Geometry check sheet. Reference: the model listing, model coordinates, mm. Face numbers are marked on the shaded views. Coordinates: 2 decimals unless noted, no trailing zeros. Loops run counter-clockwise (first coordinate to the right, second up) from the corner with the lowest first, then second, coordinate; pieces in that order, holes last. Notation, with made-up numbers: (69, -9.5) -> (76, -9.5) arc R13 ccw to (76, 2.5) -> close; hole circle Ø1 at (74.5, 63.25). An arc over 180 degrees is marked (long way). Answer as a JSON object with one key per item and string values.
from build123d import *

# Parameters (mm, degrees)
SKETCH2_W          = 5.4
SKETCH2_H          = 3.175
CUT_EXTRUDE1_DEPTH = 2
SKETCH4_R          = 2.7
CUT_EXTRUDE2_DEPTH = 3.175


with BuildPart() as part:
    # Sketch1 → Revolve3 (revolve)
    with BuildSketch(Plane(origin=(0, 0, 0), x_dir=(0, 0, -1), z_dir=(1, 0, 0))):
        with BuildLine():
            Line((4, 1.352218356), (4, 6.017854764))
            Line((4, 6.017854764), (0, 6.017854764))
            Line((0, 6.017854764), (0, -2.176614275))
            add(Edge.make_bspline(
                [(0, -2.176614275), (6.891187287, -2.176614275), (4.190169576, 0.853129288)],
                knots=[1.570796327, 1.570796327, 1.570796327, 3.544345546, 3.544345546, 3.544345546], degree=2, weights=[1, 0.551383512, 1]))
            ThreePointArc((4.190169576, 0.853129288), (4.049153077, 1.085172309), (4, 1.352218356))
        make_face()
    revolve(axis=Axis((0, 6.017854764, 0), (0, 1, 0)))

    # Sketch2 → Cut-Extrude1 (cut)
    with BuildSketch(Plane(origin=(0, 6.017854764, 0), x_dir=(1, 0, 0), z_dir=(0, 1, 0))):
        Rectangle(SKETCH2_W, SKETCH2_H)
    extrude(amount=-CUT_EXTRUDE1_DEPTH, mode=Mode.SUBTRACT)

    # Sketch4 → Cut-Extrude2 (cut)
    with BuildSketch(Plane.XY.offset(-1.5875)):
        with Locations((0, 4.017854764)):
            Circle(SKETCH4_R)
    extrude(amount=CUT_EXTRUDE2_DEPTH, mode=Mode.SUBTRACT)


solid = part.part
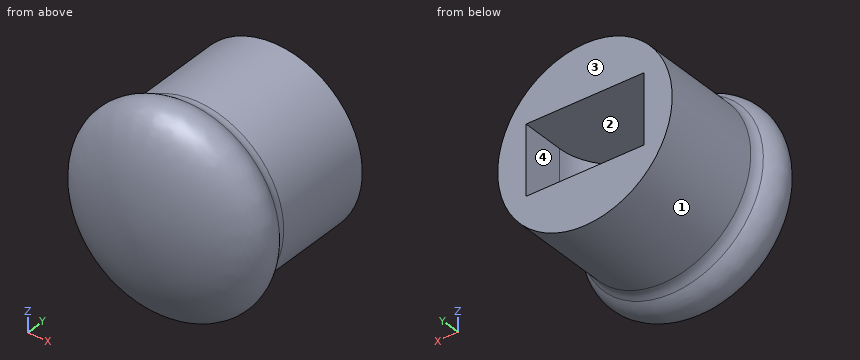
1. Section check A-A, the plane y = 2.25. Record the boundary of the cut face in (x, z), then the cut area to 3 significant figures.
Evaluation:
{"outline": "circle Ø8 at (0, 0); hole (-2.04, -1.59) -> (2.04, -1.59) -> (2.04, 1.59) -> (-2.04, 1.59) -> close", "area": "37.3 mm^2"}
2. Mould release check, pull along Z, two halves, no side actions. Record for the marked faces 1, 2, 3 and 4: released by +Z, released by -Z, zero draft, split by the parting line, or undercut.
Evaluation:
{"face 1": "split by the parting line", "face 2": "undercut", "face 3": "zero draft", "face 4": "undercut"}
3. Thickness scan on probe 1 along Z at (x, y) = (0, 1.5); probe 2 along Z at (x, y) = (-2.25, 4); probe 3 along X at (y, z) = (-1.25, -0.75). Record the ranges inside material, lowest first. Write a range as from..to.
Evaluation:
{"probe 1": "z = -4..-1.59, 1.59..4", "probe 2": "z = -3.31..-1.59, 1.59..3.31", "probe 3": "x = -3.65..3.65"}
4. Section check B-B, the plane y = 3.5. Record the boundary of the cut face in (x, z), then the cut area to 3 significant figures.
Evaluation:
{"outline": "circle Ø8 at (0, 0); hole (-2.65, -1.59) -> (2.65, -1.59) -> (2.65, 1.59) -> (-2.65, 1.59) -> close", "area": "33.4 mm^2"}
5. Depth check by flat-ended pin: P1, Ø1, axis at y = 5, z = 0.5, coming from the -X side; P2, Ø2, axis at y = 5, z = -0.5, coming from the +X side; P3, Ø2, axis at y = 1.5, z = 2, coming from the +X side; P4, Ø4, axis at x = -1.5, z = -1.5, coming from the -Y side. Enter the tip coordinate at first touch or a pass-through.
Evaluation:
{"P1": "stops at x = -4", "P2": "stops at x = 4", "P3": "stops at x = 4.09", "P4": "stops at y = -2.18"}
